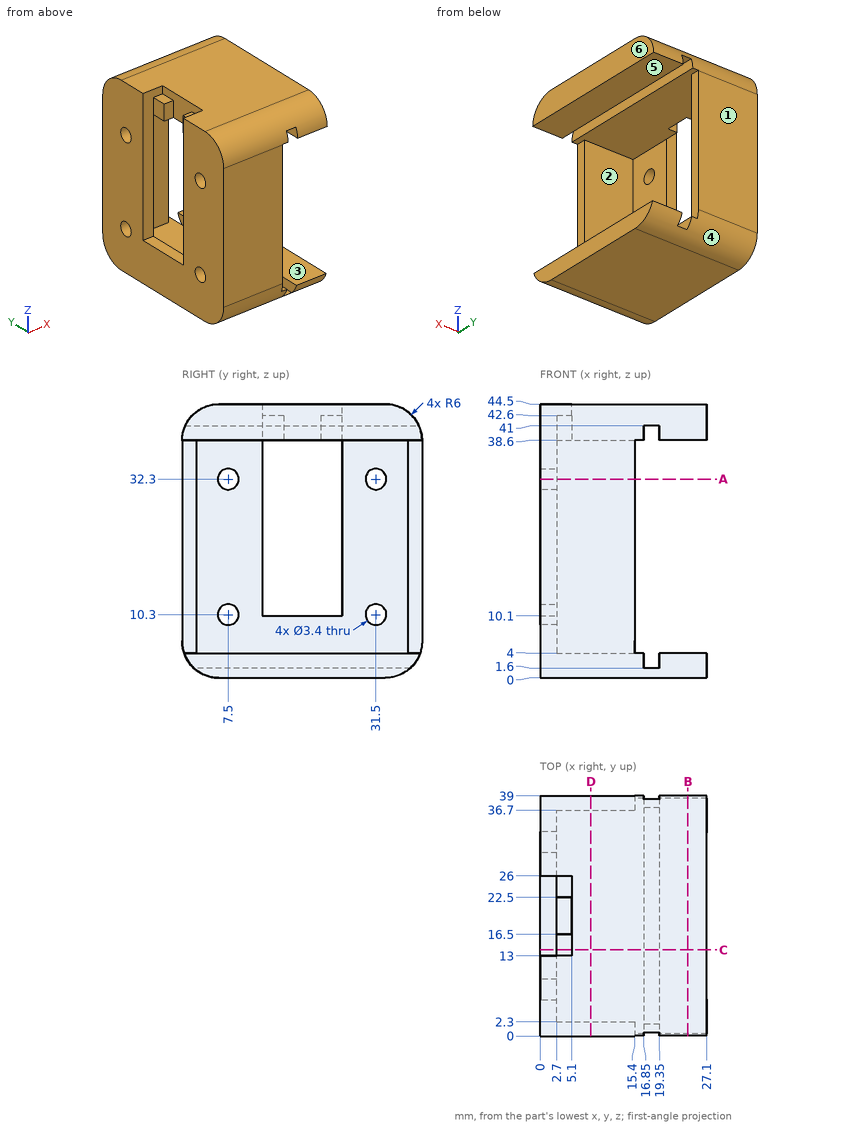
Verification items for this drawing (mm, ordinates from the low corner). A direction names the side the tool comes from. Give positions to 0.01 mm unless a question says otherwise; leave off trailing zeros. Write each loop counter-clockwise with the first axis right and the second up, starting at its lowest first coordinate (ties: lowest second). Pieces come first, ordered by that corner, then holes. Notation, with made-up numbers: (-24, -19) - (21, -19) arc R17 ccw to (21, -2) - close; hole circle Ø9 at (15, 64.25). An arc over 180 degrees is marked (long way). Answer as a JSON object with one key per item and string values. Group by question number.
1) Sectioned sample at D-D (x = 8.25). Record the cut outline in (y, z).
2) Depth check by flat-ended pin: P1, Ø3, axis at y = 31.5, z = 10.3, coming from the +X side; P2, Ø0.7, axis at y = 38, z = 27, coming from the +X side; P3, Ø2.5, axis at y = 19, z = 39.5, coming from the -X side; P4, Ø0.7, axis at x = 4, z = 40, coming from the -Y side. Enter the tip coordinate at first touch or a pass-through.
3) Sectioned sample at C-C (y = 14). Record the cut outline in (x, z).
4) Sectioned sample at A-A (z = 32.3). Record the cut outline in (x, y).
5) Thickness scan on probe 1 along Y at (x, z) = (1.05, 32.3); probe 2 along Z at (x, y) = (1.8, 31.5); probe 3 along Z at (x, y) = (11.25, 30). Record the ranges inside material, lowest first. Write a range as from..to.
6) Release check for a two-part mould opening along Z. For the marked faces 4, 5 and 6 record: pulls with the +Z half, pulls with the -Z half, needs draft (parallel to the pull), parting line crosses it, or undercut.
7) Sectioned sample at B-B (x = 24). Record the cut outline in (y, z).
8) Access from +Z, -Z, +X, -X, +Y, -Y to the whole of each face (thin tool, end or side, straight path). Record for the marked faces 1, 2 and 3.
Geometry results:
{
 "1": {"outline": "(0, 6) arc R6 ccw to (6, 0) - (33, 0) arc R6 ccw to (39, 6) - (39, 38.5) arc R6 ccw to (33, 44.5) - (6, 44.5) arc R6 ccw to (0, 38.5) - close; hole (2.3, 4) - (36.7, 4) - (36.7, 38.6) - (2.3, 38.6) - close"},
 "2": {"P1": "passes through", "P2": "stops at x = 15.4", "P3": "stops at x = 5.1", "P4": "stops at y = 0.11"},
 "3": {"outline": "(0, 0) - (27.1, 0) - (27.1, 4) - (19.35, 4) - (19.35, 1.6) - (16.85, 1.6) - (16.85, 4) - (2.7, 4) - (2.7, 10.1) - (0, 10.1) - close; (2.7, 38.6) - (16.85, 38.6) - (16.85, 41) - (19.35, 41) - (19.35, 38.6) - (27.1, 38.6) - (27.1, 44.5) - (5.1, 44.5) - (5.1, 42.6) - (2.7, 42.6) - close"},
 "4": {"outline": "(0, 0) - (15.4, 0) - (15.4, 2.3) - (2.7, 2.3) - (2.7, 5.8) - (0, 5.8) - close; (0, 9.2) - (2.7, 9.2) - (2.7, 13) - (0, 13) - close; (0, 26) - (2.7, 26) - (2.7, 29.8) - (0, 29.8) - close; (0, 33.2) - (2.7, 33.2) - (2.7, 36.7) - (15.4, 36.7) - (15.4, 39) - (0, 39) - close"},
 "5": {"probe 1": "y = 0..5.8, 9.2..13, 26..29.8, 33.2..39", "probe 2": "z = 0..8.6, 12..30.6, 34..44.5", "probe 3": "z = 0..4, 38.6..44.5"},
 "6": {"face 4": "pulls with the -Z half", "face 5": "undercut", "face 6": "needs draft"},
 "7": {"outline": "(0, 38.6) - (39, 38.6) arc R6 ccw to (33, 44.5) - (6, 44.5) arc R6 ccw to start; (0.34, 4) arc R6 ccw to (6, 0) - (33, 0) arc R6 ccw to (38.66, 4) - close"},
 "8": {"face 1": "+Z, -Z, +X, -X, +Y", "face 2": "+X", "face 3": "+X, +Y, -Y"}
}
